Work out the finished part from the listing and answer in its coordinate system (mm). Face numbers are marked on the shaded views. A direction names the side the tool comes from. Give positions to 0.01 mm unless a question says otherwise; leave off trailing zeros. Loops run counter-clockwise (first coordinate to the right, second up) from the corner with the lowest first, then second, coordinate; pieces in that order, holes last.
from build123d import *

# Parameters (mm, degrees)
F0_R     = 1.6
F0_R_2   = 0.55
F1_DEPTH = 3
F2_R     = 1


with BuildPart() as f1:
    # F0 (on Top) → F1 (new body)
    with BuildSketch(Plane.XY):
        with BuildLine():
            Line((20, 0), (20, 7.5))
            Line((20, 7.5), (17, 7.5))
            ThreePointArc((17, 7.5), (15.615652, 8.099204), (15.105048, 9.518622))
            ThreePointArc((15.105048, 9.518622), (5.125, 20.15), (-4.855048, 9.518622))
            ThreePointArc((-4.855048, 9.518622), (-5.365652, 8.099204), (-6.75, 7.5))
            Line((-6.75, 7.5), (-20, 7.5))
            Line((-20, 7.5), (-20, 0))
            Line((-20, 0), (-20, -7.5))
            Line((-20, -7.5), (20, -7.5))
            Line((20, -7.5), (20, 0))
        make_face()
        with Locations((-15, 0)):
            Circle(F0_R, mode=Mode.SUBTRACT)
        with Locations((15, 0)):
            Circle(F0_R, mode=Mode.SUBTRACT)
        with Locations((5.125, 10.15)):
            Circle(F0_R_2, mode=Mode.SUBTRACT)
    extrude(amount=F1_DEPTH)

    # F2
    f2_edges = [f1.edges().sort_by_distance(p)[0] for p in [
        (20, -7.5, 1.5),
        (20, 7.5, 1.5),
        (-20, -7.5, 1.5),
        (-20, 7.5, 1.5),
    ]]
    fillet(f2_edges, radius=F2_R)


solid = f1.part
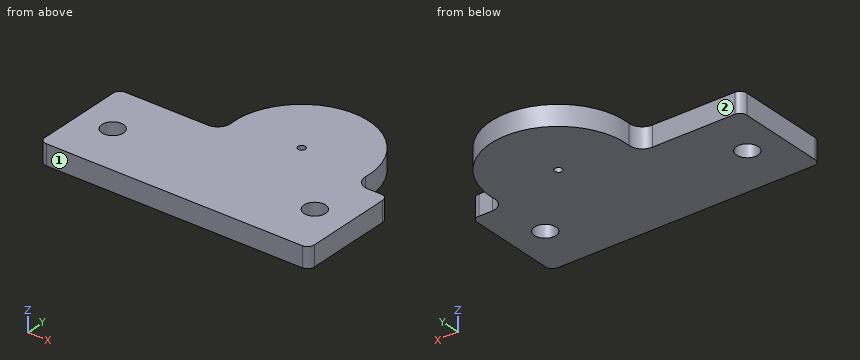
Item 1: Find section D-D, the plane z = 1.3. Write down the section's boundary in (x, y) (3 decimals).
Item 2: For the marked faces 1 and 2, determine the directions among +Z, -Z, +X, -X, +Y, -Y from which every point of the face is accessible in a straight line to the end or side of a thin tool.
Item 3: Find section B-B, the plane x = -15. Write down the section's boundary in (y, z).
Item 4: Find section A-A, the plane y = 0. Write down the section's boundary in (x, z).
Item 5: Consider line 1 (X direction, y = 0.25, z = 1.6); line 2 (Y direction, x = -15, z = 2.8); line 3 (X direction, y = 0.5, z = 1). Determine where each line is inside the solid, lowest interval first.
Item 6: Find section C-C, the plane y = 10.15. Write down the section's boundary in (x, z) (3 decimals), plus the area to 3 significant figures.
Item 7: Flat-ended cylindrical pins translate along their axes: pin 1 Ø0.9 at (x, y) = (5.125, 10.15) entering from -Z; pin 2 Ø1 at (x, z) = (18.5, 1.5) entering from +Y; pin 3 Ø1 at (y, z) = (10.5, 1) entering from +X (3 decimals). Find the tip coordinate at first contact, or state that the pin passes through.
Ans:
1. outline: (-20, -6.5) arc R1 ccw to (-19, -7.5) - (19, -7.5) arc R1 ccw to (20, -6.5) - (20, 6.5) arc R1 ccw to (19, 7.5) - (17, 7.5) arc R1.899 cw to (15.105, 9.519) arc R10 ccw (long way) to (-4.855, 9.519) arc R1.899 cw to (-6.75, 7.5) - (-19, 7.5) arc R1 ccw to (-20, 6.5) - close; hole circle Ø3.2 at (-15, 0); hole circle Ø1.1 at (5.125, 10.15); hole circle Ø3.2 at (15, 0)
2. face 1: +Z, -Z, +X, -X, -Y
2. face 2: +Z, -Z, -X, +Y
3. outline: (-7.5, 0) - (-1.6, 0) - (-1.6, 3) - (-7.5, 3) - close; (1.6, 0) - (7.5, 0) - (7.5, 3) - (1.6, 3) - close
4. outline: (-20, 0) - (-16.6, 0) - (-16.6, 3) - (-20, 3) - close; (-13.4, 0) - (13.4, 0) - (13.4, 3) - (-13.4, 3) - close; (16.6, 0) - (20, 0) - (20, 3) - (16.6, 3) - close
5. line 1: x = -20 to -16.58, -13.42 to 13.42, 16.58 to 20
5. line 2: y = -7.5 to -1.6, 1.6 to 7.5
5. line 3: x = -20 to -16.52, -13.48 to 13.48, 16.52 to 20
6. outline: (-4.875, 0) - (4.575, 0) - (4.575, 3) - (-4.875, 3) - close; (5.675, 0) - (15.125, 0) - (15.125, 3) - (5.675, 3) - close
6. area: 56.7 mm2
7. pin 1: passes through
7. pin 2: stops at y = 7.5
7. pin 3: stops at x = 15.125
